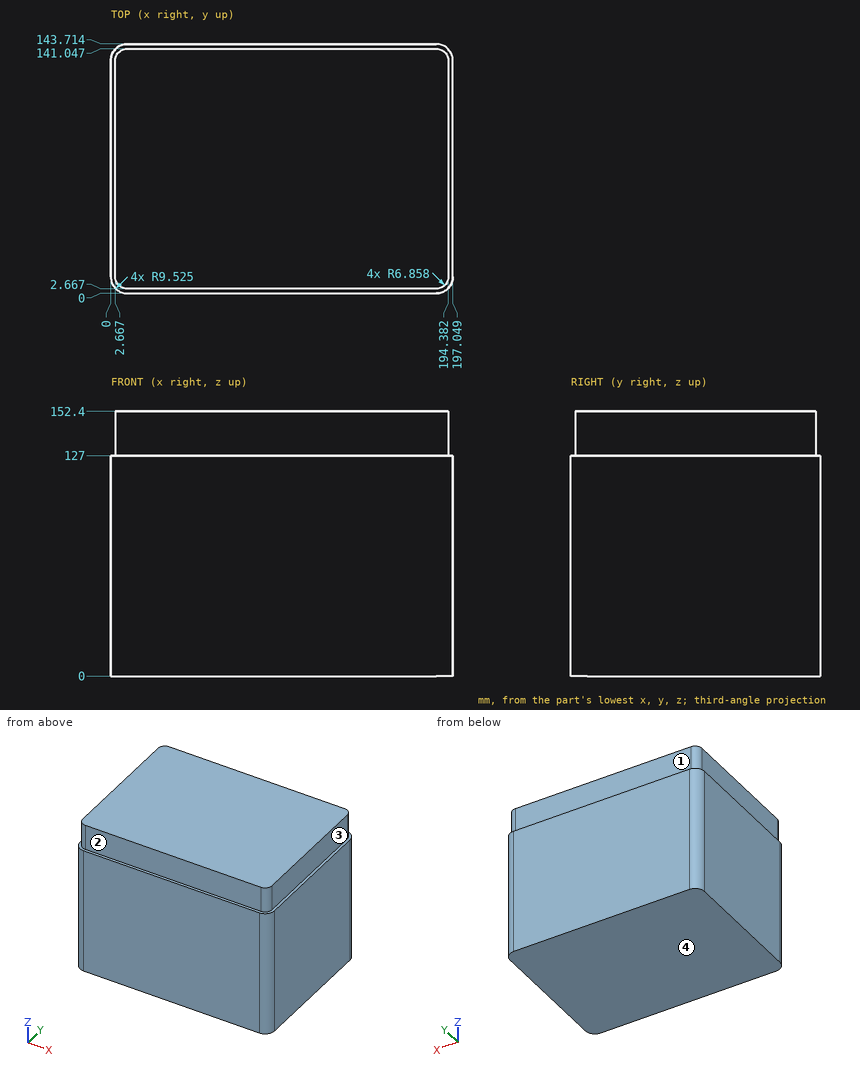
Job drawing, mm, ordinate dimensions from the low corner. One solid piece. A direction names the side the tool comes from. Give positions to 0.01 mm unless a question says otherwise; leave off trailing zeros. Answer in a Markdown table with one row per item.
1. Probe probe 1 along X at (y, z) = (21.5, 129.5); probe 2 along Y at (x, z) = (78.5, 128); probe 3 along X at (y, z) = (137, 145.5). List the from-to ranges inside material, lowest first. Write a range as [from, to].
Data:
| item | result |
|---|---|
| probe 1 | x = [2.67, 194.38] |
| probe 2 | y = [2.67, 141.05] |
| probe 3 | x = [3.27, 193.78] |
2. Tool access for the marked faces 1, 2, 3 and 4: list every direction of +Z, -Z, +X, -X, +Y, -Y with a clear straight run to the whole face (end or side of a thin tool).
Data:
| item | result |
|---|---|
| face 1 | +Z, +X, -X, +Y |
| face 2 | +Z, +X, -X, -Y |
| face 3 | +Z, +X, +Y, -Y |
| face 4 | -Z, +X, -X, +Y, -Y |
3. Flat gauge pins, fed straight in: pin 1 (1 mm diameter, centred on x = 56, z = 111, fed in from -Y); pin 2 (20.5 mm diameter, centred on y = 93, z = 138, fed in from +X); pin 3 (7.5 mm diameter, centred on x = 134.5, z = 143, fed in from +Y). Where does each tip first touch, or does it go through?
Data:
| item | result |
|---|---|
| pin 1 | stops at y = 0 |
| pin 2 | stops at x = 194.38 |
| pin 3 | stops at y = 141.05 |
